Check sheet for the modelled part. Datum: model origin and axes. Units: mm. Face numbers are marked on the shaded views. A direction names the side the tool comes from. Coordinates: 2 decimals unless noted, no trailing zeros. Loops run counter-clockwise (first coordinate to the right, second up) from the corner with the lowest first, then second, coordinate; pieces in that order, holes last. Notation, with made-up numbers: (82.5, -19.75) - (141.5, -19.75) arc R23 cw to (141.5, 17.25) - close; hole circle Ø4 at (78, -31.5). An arc over 180 degrees is marked (long way). Use a Markdown table: item, result. Add a question column.
1) Draft check along X on the marked faces 6, 7, 8 and 9. Enter one of: pulls with the +X half, pulls with the -X half, needs draft (parallel to the pull), parting line crosses it, or undercut.
2) Thickness scan on line 1 (X direction, y = -3, z = 2.25); line 2 (Z direction, x = 3.25, y = 3); line 3 (Y direction, x = 5, z = 11.5). Record the ranges inside material, lowest first.
3) Sectioned sample at A-A, the plane y = -3.5. Enter the section's corners in (x, z).
4) Go/stop test with flat-tipped pins: P1, Ø3.5, axis at y = 3, z = 1.5, coming from the +X side; P2, Ø8, axis at x = 5.5, y = 0, coming from the +Z side; P3, Ø2, axis at x = 3.5, z = 7, coming from the -Y side; P4, Ø6, axis at x = 4.5, y = 0, coming from the -Z side. Record where each tip stops, or that it passes through.
5) Sectioned sample at B-B, the plane z = 5.25. Enter the section's corners in (x, y).
6) Sectioned sample at D-D, the plane y = -10.25. Enter the section's corners in (x, z), then the cut area to 3 significant figures.
7) Sectioned sample at C-C, the plane x = 1.5. Enter the section's corners in (y, z).
8) Tool access check on the marked faces 1, 2, 3, 4 and 5. Record the directions out of +Z, -Z, +X, -X, +Y, -Y that give a thin tool (end or side, any length) a straight path to the whole face; none if there is none.
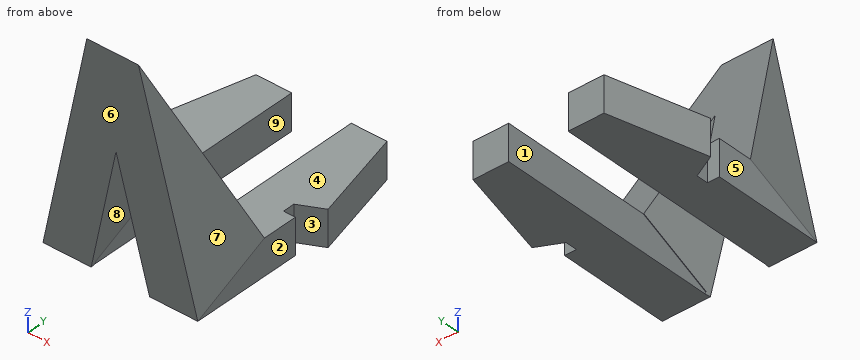
from build123d import *

# Parameters (mm, degrees)
PAD_DEPTH       = 3
POCKET_DEPTH    = 14.001
SKETCH002_W     = 13
SKETCH002_H     = 7.0986047495
PAD001_DEPTH    = 17
POCKET001_DEPTH = 14.001
POCKET002_DEPTH = 7.7802325517


with BuildPart() as part:
    # Sketch → Pad (new body)
    with BuildSketch(Plane.XY):
        Polygon((0, 0), (2, 8), (5, 8), (5, -11), (10, -11), (10, 8), (13, 8), (15, 0), (13, -1), (13, -2), (14, -2), (14, -12), (1, -12), (1, -2), (2, -2), (2, -1), align=None)
    extrude(amount=PAD_DEPTH)

    # Sketch001 (on Face4 of Pad) → Pocket (cut, through all)
    with BuildSketch(Plane.YZ.offset(14)):
        Polygon((-5, 3), (-11.4335207615, 0), (-12, 0), (-12, 3), align=None)
    extrude(amount=-POCKET_DEPTH, mode=Mode.SUBTRACT)

    # Sketch002 (on Face9 of Pocket) → Pad001 (join)
    with BuildSketch(Plane(origin=(0, -2.0420976405, 4.3792925223), x_dir=(1, 0, 0), z_dir=(0, -0.4226182617, 0.906307787))):
        with Locations((7.5, -6.8129865247)):
            Rectangle(SKETCH002_W, SKETCH002_H)
    extrude(amount=PAD001_DEPTH)

    # Sketch003 (on Face20 of Pad001) → Pocket001 (cut, through all)
    with BuildSketch(Plane.YZ.offset(14)):
        Polygon((-12.1845104496, 18.4072323796), (-11.4335207615, 0), (-18.6180312111, 15.4072323796), align=None)
    extrude(amount=-POCKET001_DEPTH, mode=Mode.SUBTRACT)

    # Sketch004 (on Face19 of Pocket001) → Pocket002 (cut, through all)
    with BuildSketch(Plane(origin=(0, -2.9579023595, -1.3792925223), x_dir=(-1, 0, 0), z_dir=(0, 0.906307787, 0.4226182617))):
        Polygon((-14, 21.8320146698), (-9.6666666667, 21.8320146698), (-14, 4.8320146698), align=None)
        Polygon((-5.3333333333, 21.8320146698), (-1, 21.8320146698), (-1, 4.8320146698), align=None)
        Polygon((-10, 4.6488008791), (-5, 4.6488008791), (-7.4999999998, 14.4564931874), align=None)
    extrude(amount=-POCKET002_DEPTH, mode=Mode.SUBTRACT)


solid = part.part
Solved:
| question | item | result |
|---|---|---|
| 1 | face 6 | needs draft |
| 1 | face 7 | pulls with the +X half |
| 1 | face 8 | undercut |
| 1 | face 9 | undercut |
| 2 | line 1 | x = 1 to 5, 10 to 14 |
| 2 | line 2 | z = 0 to 3 |
| 2 | line 3 | y = -11.9 to -8.96 |
| 3 | outline | (1, 0) - (5, 0) - (5, 3) - (1, 3) - close; (10, 0) - (14, 0) - (14, 3) - (10, 3) - close |
| 4 | P1 | stops at x = 14.69 |
| 4 | P2 | stops at z = 3 |
| 4 | P3 | stops at y = -11.76 |
| 4 | P4 | stops at z = 0 |
| 5 | outline | (1.63, -6.05) - (2.24, -11.65) - (6.28, -11.65) - (5.68, -6.05) - close; (8.72, -11.65) - (12.76, -11.65) - (13.37, -6.05) - (9.32, -6.05) - close |
| 6 | outline | (1, 0) - (5, 0) - (5, 0.55) - (5.05, 0.55) - (7.5, 11.17) - (9.95, 0.55) - (10, 0.55) - (10, 0) - (14, 0) - (14, 0.55) - (10.83, 14.26) - (4.17, 14.26) - (1, 0.55) - close |
| 6 | area | 113 mm2 |
| 7 | outline | (-11.52, 2.12) - (-11.43, 0) - (-2, 0) - (-2, 3) - (-5, 3) - (-5.83, 4.78) - close; (-0.75, 0) - (6, 0) - (6, 3) - (-0.75, 3) - close |
| 8 | face 1 | -Z, +Y |
| 8 | face 2 | +Z, -Z, +X, -Y |
| 8 | face 3 | +Z, -Z, +X |
| 8 | face 4 | +Z, +X, -X, +Y |
| 8 | face 5 | +Z, -Z, -X, -Y |
